from build123d import *

# Parameters (mm, degrees)
F1_DEPTH    = 38.1
F3_D        = 13.49248
F5_DEPTH    = 38.1
F7_DEPTH    = 38.1
F10_D       = 10.0838
F10_ON_F9_D = 10.0838


with BuildPart() as f1:
    # F0 (on Front) → F1 (new body)
    with BuildSketch(Plane.XZ):
        with BuildLine():
            Line((0, 1358.9), (0, 0))
            Line((0, 0), (990.6, 0))
            Line((990.6, 0), (990.6, 241.3))
            Line((990.6, 241.3), (864.8059485884, 1247.6524112928))
            ThreePointArc((864.8059485884, 1247.6524112928), (822.8355837767, 1327.1091283286), (738.7866582458, 1358.9))
            Line((738.7866582458, 1358.9), (0, 1358.9))
        make_face()
    extrude(amount=F1_DEPTH)

    # F3 (through all)
    with Locations(Plane.XZ.offset(38.1)):
        with Locations((698.5, 1187.45), (82.55, 914.4), (127, 1066.8), (787.4, 495.3)):
            Hole(F3_D / 2)

    # F4 (on face) → F5 (join)
    with BuildSketch(Plane(origin=(0, 0, 0), x_dir=(-1, 0, 0), z_dir=(0, 1, 0))):
        with BuildLine():
            ThreePointArc((-666.75, 1187.45), (-698.5, 1155.7), (-730.25, 1187.45))
            Line((-730.25, 1187.45), (-730.25, 1231.9))
            Line((-730.25, 1231.9), (-755.65, 1231.9))
            Line((-755.65, 1231.9), (-755.65, 1130.3))
            Line((-755.65, 1130.3), (-698.5, 1130.3))
            Line((-698.5, 1130.3), (-641.35, 1130.3))
            Line((-641.35, 1130.3), (-641.35, 1231.9))
            Line((-641.35, 1231.9), (-666.75, 1231.9))
            Line((-666.75, 1231.9), (-666.75, 1187.45))
        make_face()
    extrude(amount=F5_DEPTH)

    # F6 (on face) → F7 (join)
    with BuildSketch(Plane(origin=(0, 0, 0), x_dir=(-1, 0, 0), z_dir=(0, 1, 0))):
        with BuildLine():
            ThreePointArc((-755.65, 495.3), (-787.4, 463.55), (-819.15, 495.3))
            Line((-819.15, 495.3), (-819.15, 539.75))
            Line((-819.15, 539.75), (-844.55, 539.75))
            Line((-844.55, 539.75), (-844.55, 438.15))
            Line((-844.55, 438.15), (-787.4, 438.15))
            Line((-787.4, 438.15), (-730.25, 438.15))
            Line((-730.25, 438.15), (-730.25, 539.75))
            Line((-730.25, 539.75), (-755.65, 539.75))
            Line((-755.65, 539.75), (-755.65, 495.3))
        make_face()
    extrude(amount=F7_DEPTH)

    # F10 (through all)
    with Locations(Plane.YZ.offset(755.65)):
        with Locations((19.05, 1219.2)):
            Hole(F10_D / 2)

    # F10 on F9 (through all)
    with Locations(Plane.YZ.offset(844.55)):
        with Locations((19.05, 527.05)):
            Hole(F10_ON_F9_D / 2)


solid = f1.part
Part model, mm, in its own coordinate system. A direction names the side the tool comes from. Give positions to 0.01 mm unless a question says otherwise; leave off trailing zeros. Write each loop counter-clockwise with the first axis right and the second up, starting at its lowest first coordinate (ties: lowest second). Pieces come first, ordered by that corner, then holes.
1) Pin check, flat tips, straight feed: pin 1 (11.5 mm diameter, centred on y = 27, z = 514, fed in from +X); pin 2 (5 mm diameter, centred on y = -25, z = 544, fed in from +X) (3 decimals); pin 3 (12.5 mm diameter, centred on x = 829.5, y = 18, fed in from +Z); pin 4 (10 mm diameter, centred on x = 871.5, y = -11.5, fed in from -Z). Stop position of each tip, or through.
Resolved:
pin 1: stops at x = 844.55
pin 2: stops at x = 953.075
pin 3: stops at z = 539.75
pin 4: stops at z = 0
2) Two-plate mould, pull along Z, no slides. Class faces 5 (the face through (730.25, 19, 488)), 6 (the face through (788, 19, 438.15)), 7 (the face through (786.702, 18.783, 463.558)), 8 (the face through (743, 19, 539.75)): released by +Z, released by -Z, zero draft, split by the parting line, or undercut.
Resolved:
face 5: zero draft
face 6: released by -Z
face 7: released by +Z
face 8: undercut
3) Cut at C-C on z = 220. Write the cut outline in (x, y).
Resolved:
outline: (0, -38.1) - (990.6, -38.1) - (990.6, 0) - (0, 0) - close
4) Cut at B-B on x = 909. Write the cut outline in (y, z), then the cut area to 3 significant figures.
Resolved:
outline: (-38.1, 0) - (0, 0) - (0, 894.1) - (-38.1, 894.1) - close
area: 34,100 mm2
5) Cut at A-A on y = -16. Write the cut outline in (x, z), then the cut area to 3 significant figures.
Resolved:
outline: (0, 0) - (990.6, 0) - (990.6, 241.3) - (864.81, 1247.65) arc R127 ccw to (738.79, 1358.9) - (0, 1358.9) - close; hole circle Ø13.49 at (82.55, 914.4); hole circle Ø13.49 at (127, 1066.8); hole circle Ø13.49 at (698.5, 1187.45); hole circle Ø13.49 at (787.4, 495.3)
area: 1,260,000 mm2
6) Probe L1, parallel to Z at x = 749.5, y = 19.05; L2, parallel to Z at x = 828.75, y = 19.05; L3, parallel to Y at x = 829, z = 527. List the from-to ranges inside material, lowest first.
Resolved:
L1: z = 438.15 to 522.01, 532.09 to 539.75, 1130.3 to 1214.16, 1224.24 to 1231.9
L2: z = 438.15 to 522.01, 532.09 to 539.75
L3: y = -38.1 to 14.01, 24.09 to 38.1
7) Which spindle directions (+Z, -Z, +X, -X, +Y, -Y) get a long thin tool onto all of the face, cutting with end or side? Do faces 1 (the face through (730.25, 19, 1209)), 2 (the face through (641.35, 19, 1180)), 3 (the face through (699, 19, 1130.3)), 4 (the face through (743, 19, 1231.9)). Say none if no direction does.
Resolved:
face 1: +Z, +Y
face 2: +Z, -Z, -X, +Y
face 3: +X, -X, +Y
face 4: +Z, +X, -X, +Y
